The model under review builds one solid part; all positions refer to its coordinate system, in mm. Face numbers are marked on the shaded views. A direction names the side the tool comes from. Coordinates: 2 decimals unless noted, no trailing zeros. Loops run counter-clockwise (first coordinate to the right, second up) from the corner with the lowest first, then second, coordinate; pieces in that order, holes last. Notation, with made-up numbers: M 15.5,43.25 L 36.5,43.25 A20 ccw 36.5,61.25 Z; hole C 25,6.5 d6. An arc over 180 degrees is marked long. Use one line per item in the form item = value.
Autodesk Inventor part; units mm, degrees
ref_plane "YZ Plane" through (0, 0, 0) normal (1, 0, 0) x (0, 1, 0)
ref_plane "XZ Plane" through (0, 0, 0) normal (0, 1, 0) x (-1, 0, 0)
ref_plane "XY Plane" through (0, 0, 0) normal (0, 0, 1) x (1, 0, 0)
sketch "スケッチ1" plane through (0, 0, 0) normal (0, 0, 1) x (1, 0, 0)
  line L0 (-34.75, -10) -> (23.5151, -10) construction
  arc A0 (25, -11.4849) -> (23.5151, -10) centre (24.2575, -10.7425) ccw
  line L1 (25, -11.4849) -> (25, -13)
  line L2 (25, -13) -> (30, -13)
  line L3 (23.5151, -10) -> (25, -10) construction
  line L4 (25, -10) -> (25, -11.4849) construction
  line L5 (-34.75, -10) -> (-34.75, 42)
  line L6 (-34.75, 42) -> (43, 42)
  circle A1 centre (-13, 37) radius 1.2
  circle A2 centre (13, 37) radius 1.2
  line L7 (0, 30.2) -> (0, 0) construction
  line L8 (30, -13) -> (43, 12)
  line L9 (43, 12) -> (43, 42)
  line L10 (-22.05, 32.05) -> (33.55, 32.05)
  line L11 (33.55, 32.05) -> (33.55, 26.95)
  line L12 (33.55, 26.95) -> (-22.05, 26.95)
  line L13 (-22.05, 26.95) -> (-22.05, 32.05)
  line L14 (33.5, 32) -> (-22, 32) construction
  line L15 (-22, 32) -> (-22, 27) construction
  line L16 (-22, 27) -> (33.5, 27) construction
  line L17 (33.5, 27) -> (33.5, 32) construction
  circle A3 centre (-20, 32.05) radius 2.05
  circle A4 centre (-20, 26.95) radius 2.05
  circle A5 centre (31.5, 32.05) radius 2.05
  circle A6 centre (31.5, 26.95) radius 2.05
  line L18 (-34.75, -10) -> (-25.85, -10)
  arc A7 (-23.75, -10) -> (-25.85, -10) centre (-24.8, -10) ccw
  line L19 (-23.75, -10) -> (-23.75, -13)
  line L20 (-23.75, -13) -> (-13.75, -13)
  line L21 (-13.75, -13) -> (-13.75, -10)
  arc A8 (-11.65, -10) -> (-13.75, -10) centre (-12.7, -10) ccw
  line L22 (-11.65, -10) -> (-6.1, -10)
  arc A9 (-4, -10) -> (-6.1, -10) centre (-5.05, -10) ccw
  line L23 (-4, -10) -> (-4, -13)
  line L24 (-4, -13) -> (14, -13)
  line L25 (14, -13) -> (14, -10)
  arc A10 (16.1, -10) -> (14, -10) centre (15.05, -10) ccw
  line L26 (16.1, -10) -> (23.5151, -10)
  line L27 (18.45, -6.1712) -> (21.55, -6.1712) construction
  line L28 (21.55, -6.1712) -> (21.55, -12.9737) construction
  line L29 (21.55, -12.9737) -> (18.45, -12.9737) construction
  line L30 (18.45, -12.9737) -> (18.45, -6.1712) construction
  line L31 (-31.3, -5.7897) -> (-28.2, -5.7897) construction
  line L32 (-28.2, -5.7897) -> (-28.2, -15) construction
  line L33 (-28.2, -15) -> (-31.3, -15) construction
  line L34 (-31.3, -15) -> (-31.3, -5.7897) construction
  line L35 (-29.75, -5.7897) -> (-29.75, -15) construction
  line L36 (20, -6.1712) -> (20, -12.9737) construction
  line L37 (43, 42) -> (55.5, 38.3823)
  line L38 (55.5, 38.3823) -> (55.5, 15.6177)
  line L39 (55.5, 15.6177) -> (43, 12)
  circle A11 centre (51, 35) radius 1.55
  circle A12 centre (51, 19) radius 1.55
  circle A13 centre (51, 35) radius 4.5 construction
  circle A14 centre (51, 19) radius 4.5 construction
  line L40 (51, 35) -> (51, 19) construction
  line L41 (-11.2651, 33.995) -> (-14.7349, 33.995)
  line L42 (-14.7349, 33.995) -> (-16.4699, 37)
  line L43 (-16.4699, 37) -> (-14.7349, 40.005)
  line L44 (-14.7349, 40.005) -> (-11.2651, 40.005)
  line L45 (-11.2651, 40.005) -> (-9.5301, 37)
  line L46 (-9.5301, 37) -> (-11.2651, 33.995)
  circle A15 centre (-15.4199, 37) radius 1.05
  circle A16 centre (-14.2099, 34.9043) radius 1.05
  circle A17 centre (-11.7901, 34.9043) radius 1.05
  circle A18 centre (-10.5801, 37) radius 1.05
  circle A19 centre (-11.7901, 39.0957) radius 1.05
  circle A20 centre (-14.2099, 39.0957) radius 1.05
  line L47 (16.4699, 37) -> (14.7349, 33.995)
  line L48 (14.7349, 33.995) -> (11.2651, 33.995)
  line L49 (11.2651, 33.995) -> (9.5301, 37)
  line L50 (9.5301, 37) -> (11.2651, 40.005)
  line L51 (11.2651, 40.005) -> (14.7349, 40.005)
  line L52 (14.7349, 40.005) -> (16.4699, 37)
  circle A21 centre (10.5801, 37) radius 1.05
  circle A22 centre (11.7901, 34.9043) radius 1.05
  circle A23 centre (14.2099, 34.9043) radius 1.05
  circle A24 centre (15.4199, 37) radius 1.05
  circle A25 centre (14.2099, 39.0957) radius 1.05
  circle A26 centre (11.7901, 39.0957) radius 1.05
  line L53 (1.7349, 33.995) -> (-1.7349, 33.995)
  line L54 (-1.7349, 33.995) -> (-3.4699, 37)
  line L55 (-3.4699, 37) -> (-1.7349, 40.005)
  line L56 (-1.7349, 40.005) -> (1.7349, 40.005)
  line L57 (1.7349, 40.005) -> (3.4699, 37)
  line L58 (3.4699, 37) -> (1.7349, 33.995)
  circle A27 centre (-2.4199, 37) radius 1.05
  circle A28 centre (-1.2099, 34.9043) radius 1.05
  circle A29 centre (1.2099, 34.9043) radius 1.05
  circle A30 centre (2.4199, 37) radius 1.05
  circle A31 centre (1.2099, 39.0957) radius 1.05
  circle A32 centre (-1.2099, 39.0957) radius 1.05
  line L59 (51, 38.1754) -> (53.75, 36.5877)
  line L60 (53.75, 36.5877) -> (53.75, 33.4123)
  line L61 (53.75, 33.4123) -> (51, 31.8246)
  line L62 (51, 31.8246) -> (48.25, 33.4123)
  line L63 (48.25, 33.4123) -> (48.25, 36.5877)
  line L64 (48.25, 36.5877) -> (51, 38.1754)
  point P0 (43, 27)
  point P1 (55.5, 27)
  point P2 (-14.7349, 33.995)
  point P3 (-11.2651, 33.995)
  point P4 (-9.5301, 37)
  point P5 (-11.2651, 40.005)
  point P6 (-14.7349, 40.005)
  point P7 (14.7349, 40.005)
  point P8 (11.2651, 40.005)
  point P9 (0, 37)
  point P10 (3.4699, 37)
  point P11 (1.7349, 40.005)
  point P12 (-1.7349, 40.005)
  dimension "d110" = 4.1
  dimension "d201" = 2.1
  dimension "d42" = 2.4
  dimension "d44" = 13
  dimension "d90" = 5
  dimension "d91" = 59.75
  dimension "d92" = 1.05
  dimension "d93" = 25
  dimension "d95" = 3
  dimension "d96" = 10
  dimension "d97" = 43
  dimension "d98" = 30
  dimension "d99" = 52
  dimension "d100" = 37
  dimension "d104" = 55.5
  dimension "d105" = 0.05
  dimension "d106" = 22
  dimension "d107" = 42
  dimension "d109" = 5
  dimension "d111" = 1.05
  dimension "d113" = 49.75
  dimension "d114" = 5
  dimension "d115" = 3.1
  dimension "d116" = 6
  dimension "d117" = 6
  dimension "d118" = 10
  dimension "d119" = 18
  dimension "d120" = 3
  dimension "d184" = 3.1
  dimension "d186" = 16
  dimension "d200" = 6.01
  dimension "d204" = 360
  dimension "d208" = 360
  dimension "d212" = 360
  dimension "d214" = 13
  dimension "d216" = 5.5
  dimension "d217" = 9
  dimension "d218" = 8
extrude "押し出し1" add sketch "スケッチ1" along normal blind 5 contours A0 L26 A10 L25 L24 L23 A9 L22 A8 L21 L20 L19 A7 L18 L5 L6 L9 L8 L2 L1 | L9 L37 L38 L39 | A1 | A2 | A17 L41 | L41 A17 L46 | L46 A17 | L41 A16 L42 A15 L43 A20 L44 A19 L45 A18 L46 A17 | A16 L41 | L41 L42 A16 | A18 L45 L46 | L46 A18 | A16 L42 | L45 A18 | A19 L44 L45 | L45 A19 | A15 L42 | L42 L43 A15 | L44 A19 | A15 L43 | A20 L43 L44 | L44 A20 | L43 A20 | A23 L47 | A23 L48 A22 L49 A21 L50 A26 L51 A25 L52 A24 L47 | L47 L48 A23 | A23 L48 | A24 L52 L47 | L47 A24 | L52 A24 | A22 L48 | L48 L49 A22 | A25 L51 L52 | L52 A25 | A22 L49 | L51 A25 | A26 L50 L51 | L51 A26 | A21 L49 | L49 L50 A21 | L50 A26 | A21 L50 | A29 L53 | L53 A29 L58 | L58 A29 | L53 A28 L54 A27 L55 A32 L56 A31 L57 A30 L58 A29 | A28 L53 | L53 L54 A28 | A30 L57 L58 | L58 A30 | A28 L54 | L57 A30 | A31 L56 L57 | L57 A31 | A27 L54 | L54 L55 A27 | L56 A31 | A27 L55 | A32 L55 L56 | L56 A32 | L55 A32 | L59 L60 L61 L62 L63 L64
sketch "スケッチ9" plane through (0, 0, 0) normal (0, 0, -1) x (-1, 0, 0)
  line L0 (-16.1, -10) -> (-23.5151, -10)
  line L1 (17.95, 26.95) -> (-29.45, 26.95)
  arc A0 (-33.55, 26.95) -> (-29.45, 26.95) centre (-31.5, 26.95) ccw
  line L2 (-33.55, 26.95) -> (-33.55, 32.05)
  arc A1 (-29.45, 32.05) -> (-33.55, 32.05) centre (-31.5, 32.05) ccw
  line L3 (-29.45, 32.05) -> (17.95, 32.05)
  arc A2 (22.05, 32.05) -> (17.95, 32.05) centre (20, 32.05) ccw
  line L4 (22.05, 32.05) -> (22.05, 26.95)
  arc A3 (17.95, 26.95) -> (22.05, 26.95) centre (20, 26.95) ccw
  circle A4 centre (-10, 36) radius 1.2
  circle A5 centre (10, 36) radius 1.2
  circle A6 centre (-51, 19) radius 1.55
  circle A7 centre (-51, 35) radius 1.55
  line L5 (-67.988, 57.9937) -> (81.7485, 57.9937)
  line L6 (81.7485, 57.9937) -> (81.7485, -5)
  line L7 (81.7485, -5) -> (-67.988, -5)
  line L8 (-67.988, -5) -> (-67.988, 57.9937)
  point P0 (0, 0)
  dimension "d197" = 5
extrude "押し出し5" cut sketch "スケッチ9" against normal blind 2 contours A4 | A5 | L5 L6 L7 L8
sketch "スケッチ12" plane through (0, 0, 5) normal (0, 0, 1) x (1, 0, 0)
  circle A0 centre (51, 35) radius 1.55
  circle A1 centre (51, 35) radius 1.55
  circle A2 centre (51, 27) radius 3
  circle A3 centre (51, 27) radius 3
  circle A4 centre (51, 19) radius 1.55
  circle A5 centre (51, 19) radius 1.55
  point P0 (0, 0)
extrude "押し出し8" add sketch "スケッチ12" against normal up to surface (3 mm away)
equation "\"d91\" = d54"
properties part number "胴体_サブフレーム_1_1" material "アルミニウム 2014-T4"
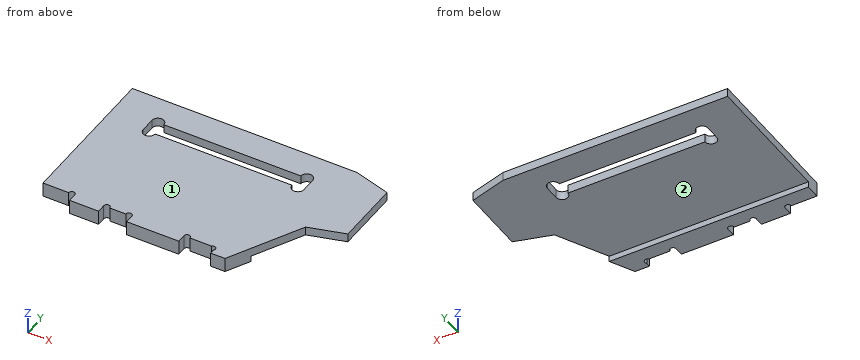
1. Wall thickness on line 1 along Y through (x, z) = (-3, 4.25); line 2 along Y through (x, z) = (-10, 4); line 3 along Z through (x, y) = (-1, 22.5): over which ranges is each line inside the solid? List them lowest first. Write a range as from..to.
Response values:
line_1 = -13..26.95, 32.05..42
line_2 = -10..26.95, 32.05..42
line_3 = 2..5
2. Add section B-B (y = 28.5). State the section outline as (x, z) points, then the cut area to 3 significant figures.
Response values:
outline = M -34.75,2 L -22.05,2 L -22.05,5 L -34.75,5 Z; M 33.55,2 L 55.5,2 L 55.5,5 L 33.55,5 Z
area = 104 mm^2
3. Add section D-D (x = -24.8). State the section outline as (y, z) points.
Response values:
outline = M -8.95,0 L -5,0 L -5,2 L 42,2 L 42,5 L -8.95,5 Z
4. Insertion check: P1, Ø0.6, axis at x = -12, z = 0.5, coming from the +Y side; P2, Ø2.5, axis at x = -32, z = 3, coming from the -Y side; P3, Ø1.2, axis at y = -12.5, z = 1.5, coming from the -X side. Each pin has a flat end and moves straight along its axis. Give the tip position at first contact, or say it passes through.
Response values:
P1 = -5
P2 = -10
P3 = -23.75
5. Machinability: for the marked faces 1 and 2, which of the approach directions +Z, -Z, +X, -X, +Y, -Y give a long, thin tool a straight path to every point of the face, cutting with its end or side? Answer none if there is none.
Response values:
face_1 = +Z, +X, -X, +Y, -Y
face_2 = -Z, +X, -X, +Y
6. Add section A-A (x = 15.05). State the section outline as (y, z) points.
Response values:
outline = M -8.95,0 L -5,0 L -5,2 L 26.95,2 L 26.95,5 L -8.95,5 Z; M 32.05,2 L 42,2 L 42,5 L 32.05,5 Z
